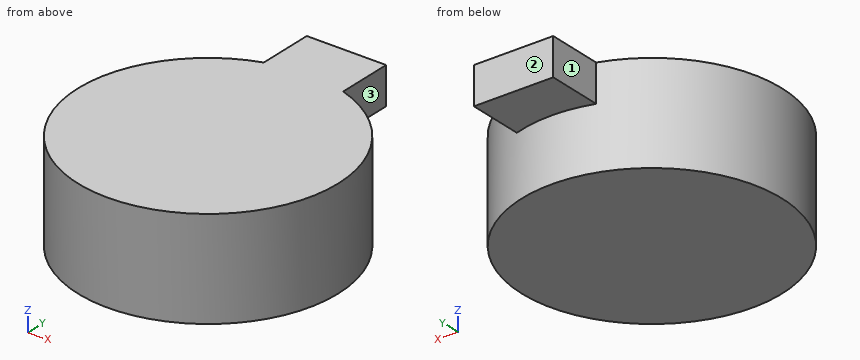
```python
from build123d import *

# Parameters (mm, degrees)
SKIZZE1_R                       = 5.25
AUFSATZ_LINEAR_AUSTRAGEN1_DEPTH = 4
SKIZZE2_W                       = 3.2
SKIZZE2_H                       = 7.25
AUFSATZ_LINEAR_AUSTRAGEN2_DEPTH = 1.5


with BuildPart() as part:
    # Skizze1 → Aufsatz-Linear austragen1 (new body)
    with BuildSketch(Plane.XY):
        with Locations((-117.143982167, 15.456381225)):
            Circle(SKIZZE1_R)
    extrude(amount=-AUFSATZ_LINEAR_AUSTRAGEN1_DEPTH)

    # Skizze2 → Aufsatz-Linear austragen2 (add)
    with BuildSketch(Plane.XY):
        with Locations((-117.143982167, 19.081381225)):
            Rectangle(SKIZZE2_W, SKIZZE2_H)
    extrude(amount=-AUFSATZ_LINEAR_AUSTRAGEN2_DEPTH)


solid = part.part
```
Input: part model. Units: mm. Frame: model coordinates. Face numbers are marked on the shaded views. A direction names the side the tool comes from. Coordinates: 2 decimals unless noted, no trailing zeros. Write each loop counter-clockwise with the first axis right and the second up, starting at its lowest first coordinate (ties: lowest second). Pieces come first, ordered by that corner, then holes.
1) Section B-B on x = -115.75. Output: boundary loops of the cut face in (y, z).
2) Section D-D on x = -118.5. Output: boundary loops of the cut face in (y, z).
3) Material intervals for line 1 along Z through (x, y) = (-115.75, 21.25); line 2 along X through (y, z) = (14.75, -2.7); line 3 along X through (y, z) = (12.5, -0.9), sorted ascending.
4) Section C-C on y = 12.5. Output: boundary loops of the cut face in (x, z), and give its area (3 significant figures).
5) Pin query (flat end, axial travel): pin 1 Ø2 at (x, z) = (-120, -1.5) entering from -Y; pin 2 Ø1.1 at (x, y) = (-117.5, 21.5) entering from -Z. Return the tip coordinate at first contact, or that it passes through.
6) Set-up query: the marked faces 1, 2 and 3. Return all of +Z, -Z, +X, -X, +Y, -Y with unobstructed straight access to the full face (end or side cutting, diameter ignored); none if empty.
7) Section A-A on z = -1.2. Output: boundary loops of the cut face in (x, y), and give its area (3 significant figures).
Check result:
1. outline: (10.39, -4) - (20.52, -4) - (20.52, -1.5) - (22.71, -1.5) - (22.71, 0) - (10.39, 0) - close
2. outline: (10.38, -4) - (20.53, -4) - (20.53, -1.5) - (22.71, -1.5) - (22.71, 0) - (10.38, 0) - close
3. line 1: z = -1.5 to 0
3. line 2: x = -122.35 to -111.94
3. line 3: x = -121.48 to -112.81
4. outline: (-121.48, -4) - (-112.81, -4) - (-112.81, 0) - (-121.48, 0) - close
4. area: 34.7 mm2
5. pin 1: stops at y = 10.55
5. pin 2: stops at z = -1.5
6. face 1: +Z, -Z, -X, +Y
6. face 2: +Z, -Z, +X, -X, +Y
6. face 3: +Z, -Z, +X, +Y
7. outline: (-118.74, 20.46) arc R5.25 ccw (long way) to (-115.54, 20.46) - (-115.54, 22.71) - (-118.74, 22.71) - close
7. area: 93.3 mm2
